```python
from build123d import *

# Parameters (mm, degrees)
SKETCH_1_R          = 3
EXTRUDE_1_DEPTH     = 19.4
SKETCH_2_W          = 20
SKETCH_2_H          = 13
CUT_EXTRUDE_1_DEPTH = 68.47303165


with BuildPart() as part:
    # 草图1 → 凸台-拉伸1 (new body)
    with BuildSketch(Plane.XY):
        with BuildLine():
            Line((-57.5, 6), (57.5, 6))
            ThreePointArc((57.5, 6), (63.5, 0), (57.5, -6))
            Line((57.5, -6), (-57.5, -6))
            ThreePointArc((-57.5, -6), (-63.5, 0), (-57.5, 6))
        make_face()
        with Locations((-57.5, 0)):
            Circle(SKETCH_1_R, mode=Mode.SUBTRACT)
        with Locations((57.5, 0)):
            Circle(SKETCH_1_R, mode=Mode.SUBTRACT)
    extrude(amount=EXTRUDE_1_DEPTH)

    # 草图2 → 切除-拉伸1 (cut, through all)
    with BuildSketch(Plane(origin=(0, 6, 0), x_dir=(1, 0, 0), z_dir=(0, 1, 0))):
        with Locations((-53.5, -9.7)):
            Rectangle(SKETCH_2_W, SKETCH_2_H)
        with Locations((53.5, -9.7)):
            Rectangle(SKETCH_2_W, SKETCH_2_H)
        with BuildLine():
            Line((-34.8, -3.2), (34.8, -3.2))
            ThreePointArc((34.8, -3.2), (36.709188309, -3.990811691), (37.5, -5.9))
            Line((37.5, -5.9), (37.5, -13.5))
            ThreePointArc((37.5, -13.5), (36.709188309, -15.409188309), (34.8, -16.2))
            Line((34.8, -16.2), (-34.8, -16.2))
            ThreePointArc((-34.8, -16.2), (-36.709188309, -15.409188309), (-37.5, -13.5))
            Line((-37.5, -13.5), (-37.5, -5.9))
            ThreePointArc((-37.5, -5.9), (-36.709188309, -3.990811691), (-34.8, -3.2))
        make_face()
    extrude(amount=-CUT_EXTRUDE_1_DEPTH, mode=Mode.SUBTRACT)


solid = part.part
```
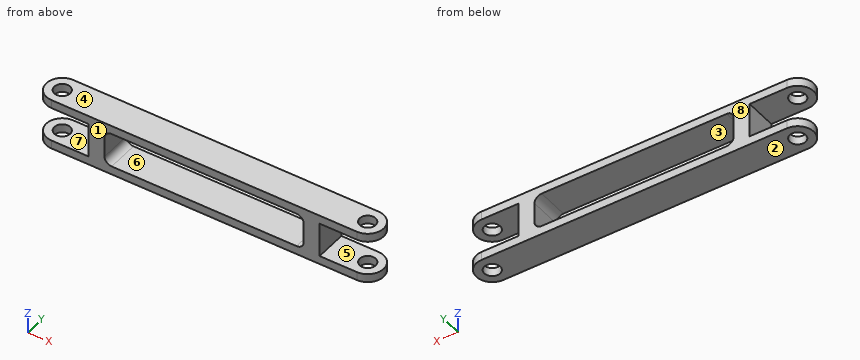
Check sheet for the modelled part. Datum: model origin and axes. Units: mm. Face numbers are marked on the shaded views. A direction names the side the tool comes from. Round coordinates to 2 decimals unless told otherwise and drop trailing zeros. Write each loop counter-clockwise with the first axis right and the second up, starting at its lowest first coordinate (ties: lowest second). Pieces come first, ordered by that corner, then holes. Notation, with made-up numbers: (38, -18) -> (90, -18) arc R16 ccw to (90, -5) -> close; hole circle Ø8 at (27, 85.25). An arc over 180 degrees is marked (long way). Put each result on its own line as item: value.
(1) Material ranges on line 1 (X direction, y = 0, z = 17.5); line 2 (Y direction, x = 57.5, z = 16.95); line 3 (Z direction, x = 51, y = -1.25), recorded low to high.
Values found:
line 1: x = -63.5 to -60.5, -54.5 to 54.5, 60.5 to 63.5
line 2: y = -6 to -3, 3 to 6
line 3: z = 0 to 3.2, 16.2 to 19.4
(2) Sectioned sample at D-D (z = 4.5). Enter the section's corners in (x, y).
Values found:
outline: (-43.5, -6) -> (-37.11, -6) -> (-37.11, 6) -> (-43.5, 6) -> close; (37.11, -6) -> (43.5, -6) -> (43.5, 6) -> (37.11, 6) -> close
(3) Mould release check, pull along Z, two halves, no side actions. Record for the marked faces 1, 2, 3 and 4: released by +Z, released by -Z, zero draft, split by the parting line, or undercut.
Values found:
face 1: zero draft
face 2: released by -Z
face 3: undercut
face 4: released by +Z
(4) Sectioned sample at A-A (x = 21). Enter the section's corners in (y, z), plus the area to 3 significant figures.
Values found:
outline: (-6, 0) -> (6, 0) -> (6, 3.2) -> (-6, 3.2) -> close; (-6, 16.2) -> (6, 16.2) -> (6, 19.4) -> (-6, 19.4) -> close
area: 76.8 mm^2
(5) Go/stop test with flat-tipped pins: pin 1 Ø2.5 at (y, z) = (1.5, 9.5) entering from +X; pin 2 Ø2.5 at (y, z) = (-2, 8.5) entering from -X. Record where each tip stops, or that it passes through.
Values found:
pin 1: stops at x = 43.5
pin 2: stops at x = -43.5
(6) Tool access check on the marked faces 5, 6, 7 and 8. Record the directions out of +Z, -Z, +X, -X, +Y, -Y that give a thin tool (end or side, any length) a straight path to the whole face; none if there is none.
Values found:
face 5: +X, +Y, -Y
face 6: +Y, -Y
face 7: -X, +Y, -Y
face 8: +Z, -Z, +X, -X, +Y
(7) Sectioned sample at B-B (y = 0). Count the separate pieces of the cut face and the enclosed holes in it, plus the area to 3 significant figures.
Values found:
separate pieces: 5
enclosed holes: 1
area: 898 mm^2
(8) Sectioned sample at C-C (z = 18). Enter the section's corners in (x, y).
Values found:
outline: (-57.5, -6) -> (57.5, -6) arc R6 ccw to (57.5, 6) -> (-57.5, 6) arc R6 ccw to start; hole circle Ø6 at (-57.5, 0); hole circle Ø6 at (57.5, 0)
